Verification items for the finished model (mm, model axes). A direction names the side the tool comes from. Coordinates: 2 decimals unless noted, no trailing zeros. Write each loop counter-clockwise with the first axis right and the second up, starting at its lowest first coordinate (ties: lowest second). Pieces come first, ordered by that corner, then holes. Notation, with made-up numbers: M 49,-13.75 L 64,-13.75 A34 cw 64,21.25 Z; hole C 66,16.25 d3. An arc over 180 degrees is marked long. Answer in a Markdown table with one row per item.
from build123d import *

# Parameters (mm, degrees)
BOX_W           = 37
BOX_H           = 39
BOX_DEPTH       = 14
SKETCH_W        = 26
SKETCH_H        = 32
POCKET_DEPTH    = 15
SKETCH001_W     = 2.3
SKETCH001_H     = 8.3
POCKET001_DEPTH = 34
SKETCH002_W     = 39
SKETCH002_H     = 14
PAD001_DEPTH    = 2


with BuildPart() as part:
    # Box → Box (new body)
    with BuildSketch(Plane(origin=(-14, -33, -31), x_dir=(1, 0, 0), z_dir=(0, 0, 1))):
        with Locations((18.5, 19.5)):
            Rectangle(BOX_W, BOX_H)
    extrude(amount=BOX_DEPTH)

    # Sketch → Pocket (cut)
    with BuildSketch(Plane(origin=(-14, -33, -31), x_dir=(1, 0, 0), z_dir=(0, 0, -1))):
        with Locations((19, -23)):
            Rectangle(SKETCH_W, SKETCH_H)
    extrude(amount=-POCKET_DEPTH, mode=Mode.SUBTRACT)

    # Sketch001 → Pocket001 (cut)
    with BuildSketch(Plane(origin=(-14, 6, -31), x_dir=(-1, 0, 0), z_dir=(0, 1, 0))):
        with Locations((-35.75, 7.064953)):
            Rectangle(SKETCH001_W, SKETCH001_H)
    extrude(amount=-POCKET001_DEPTH, mode=Mode.SUBTRACT)

    # Sketch002 → Pad001 (new body)
    with BuildSketch(Plane(origin=(23, -33, -31), x_dir=(0, 1, 0), z_dir=(1, 0, 0))):
        with Locations((19.5, 7)):
            Rectangle(SKETCH002_W, SKETCH002_H)
    extrude(amount=PAD001_DEPTH)


solid = part.part
1) Sectioned sample at D-D (z = -23). Record the cut outline in (x, y).
Response values:
| item | result |
|---|---|
| outline | M -14,-33 L 25,-33 L 25,6 L 22.9,6 L 22.9,-28 L 20.6,-28 L 20.6,6 L 18,6 L 18,-26 L -8,-26 L -8,6 L -14,6 Z |
2) Tool access check on faces 4 (the face through (-8, -10, -24)), 5 (the face through (25, -14, -24)), 6 (the face through (20.6, -11, -24)). Record the directions out of +Z, -Z, +X, -X, +Y, -Y that give a thin tool (end or side, any length) a straight path to the whole face; none if there is none.
Response values:
| item | result |
|---|---|
| face 4 | +Z, -Z, +Y |
| face 5 | +Z, -Z, +X, +Y, -Y |
| face 6 | +Y |
3) Sectioned sample at B-B (z = -19). Record the cut outline in (x, y).
Response values:
| item | result |
|---|---|
| outline | M -14,-33 L 25,-33 L 25,6 L 18,6 L 18,-26 L -8,-26 L -8,6 L -14,6 Z |
4) Release check for a two-part mould opening along X. For faces 1 (the face through (-11, 6, -24)), 2 (the face through (-14, -14, -24)), 3 (the face through (5, -26, -24)) record: +X half, -X half, draft (parallel to the pull), parting line (faces both ways), or undercut.
Response values:
| item | result |
|---|---|
| face 1 | draft |
| face 2 | -X half |
| face 3 | undercut |
5) Sectioned sample at A-A (y = -8.5). Record the cut outline in (x, z), then the cut area to 3 significant figures.
Response values:
| item | result |
|---|---|
| outline | M -14,-31 L -8,-31 L -8,-17 L -14,-17 Z; M 18,-31 L 25,-31 L 25,-17 L 18,-17 Z; hole M 20.6,-28.09 L 22.9,-28.09 L 22.9,-19.79 L 20.6,-19.79 Z |
| area | 163 mm² |
6) Sectioned sample at C-C (x = 22). Record the cut outline in (y, z), then the cut area to 3 significant figures.
Response values:
| item | result |
|---|---|
| outline | M -33,-31 L 6,-31 L 6,-28.09 L -28,-28.09 L -28,-19.79 L 6,-19.79 L 6,-17 L -33,-17 Z |
| area | 264 mm² |
7) Thickness scan on L1, parallel to X at y = -7, z = -25; L2, parallel to X at y = -8.5, z = -19.75; L3, parallel to Y at x = 12.5, z = -18.25. Record the ranges inside material, lowest first. Write a range as [from, to].
Response values:
| item | result |
|---|---|
| L1 | x = [-14, -8], [18, 20.6], [22.9, 25] |
| L2 | x = [-14, -8], [18, 25] |
| L3 | y = [-33, -26] |
8) Depth check by flat-ended pin: pin 1 (7 mm diameter, centred on x = 1, z = -22.5, fed in from +Y). Enter the tip coordinate at first touch or a pass-through.
Response values:
| item | result |
|---|---|
| pin 1 | stops at y = -26 |
